from build123d import *

# Parameters (mm, degrees)
SKETCH_1_R      = 4
EXTRUDE_1_DEPTH = 13
SKETCH_2_W      = 0.5
SKETCH_2_H      = 0.5
EXTRUDE_2_DEPTH = 1
SKETCH_3_W      = 0.5
SKETCH_3_H      = 0.5
EXTRUDE_3_DEPTH = 5.5
FILLET_1_R      = 0.25
FILLET_2_R      = 0.25


with BuildPart() as part:
    # Эскиз1 → Бобышка-Вытянуть1 (new body)
    with BuildSketch(Plane.XY):
        with Locations(Location((0, 0, 0), (0, 0, 180))):
            Circle(SKETCH_1_R)
    extrude(amount=EXTRUDE_1_DEPTH)

    # Эскиз2 → Бобышка-Вытянуть2 (add)
    with BuildSketch(Plane(origin=(0, 0, 0), x_dir=(-1, 0, 0), z_dir=(0, 0, -1))):
        with Locations((2, 0)):
            Rectangle(SKETCH_2_W, SKETCH_2_H)
        with Locations((-2, 0)):
            Rectangle(SKETCH_2_W, SKETCH_2_H)
    extrude(amount=EXTRUDE_2_DEPTH)

    # Эскиз3 → Бобышка-Вытянуть3 (add)
    with BuildSketch(Plane.XZ.offset(0.25)):
        with Locations((-2, -0.75)):
            Rectangle(SKETCH_3_W, SKETCH_3_H)
        with Locations((2, -0.75)):
            Rectangle(SKETCH_3_W, SKETCH_3_H)
    extrude(amount=EXTRUDE_3_DEPTH)

    # Скругление1
    fillet_1_edges = [part.edges().sort_by_distance(p)[0] for p in [
        (-1.75, -2.75, -1),
        (-2.25, -2.75, -1),
    ]]
    fillet(fillet_1_edges, radius=FILLET_1_R - 0.0001)  # a hair under: the kernel refuses the full size

    # Скругление2
    fillet_2_edges = [part.edges().sort_by_distance(p)[0] for p in [
        (-1.75, -0.25, -0.25),
        (-2.25, -0.25, -0.25),
        (-2.25, -3, -0.5),
        (-2, -0.25, -0.5),
        (-1.75, -3, -0.5),
        (1.75, -0.25, -0.25),
        (2.25, -0.25, -0.25),
        (1.75, -3, -0.5),
        (2, -0.25, -0.5),
        (2.25, -3, -0.5),
        (-1.75, 0.25, -0.37505),
        (-2.25, 0.25, -0.37505),
        (-2.176805985, 0.25, -0.926805985),
        (-1.823194015, 0.25, -0.926805985),
        (1.75, 0.25, -0.5),
        (2.25, 0.25, -0.5),
        (1.75, -2.75, -1),
        (2, 0.25, -1),
        (2.25, -2.75, -1),
    ]]
    fillet(fillet_2_edges, radius=FILLET_2_R - 0.0001)  # a hair under: the kernel refuses the full size


solid = part.part
Could you check a few things on this model? Use its own coordinates, in mm. Coordinates: 2 decimals unless noted, no trailing zeros. Write each loop counter-clockwise with the first axis right and the second up, starting at its lowest first coordinate (ties: lowest second). Pieces come first, ordered by that corner, then holes. Notation, with made-up numbers: (-28.5, 7.25) - (16.5, 7.25) arc R18 cw to (16.5, 23.25) - close; hole circle Ø2 at (4, 56). An arc over 180 degrees is marked (long way). Put each result on its own line as item: value. Start each with the question number.
Q1. I'm going to push flat-ended pins straight in: P1, Ø2, axis at x = 0.5, y = -1.5, coming from the -Z side; P2, Ø1.5, axis at y = 1.5, z = 5.5, coming from the -X side; P3, Ø3, axis at x = -2, z = 10, coming from the +Y side. Where does each tip first touch, or does it pass through?
Q2. I want a section at B-B on z = 2. Write out the boundary of the cut face in (x, y).
Q3. I want a section at A-A on y = -2.25. Count the separate pieces of the cut face and the enclosed holes in it, plus the area to 3 significant figures.
Q4. Please list where these lines run through material, in increasing order: L1, parallel to Z at x = -2, y = 2.5; L2, parallel to Y at x = 0, z = 12.25; L3, parallel to Y at x = -2.25, z = 5.25.
Q5. I want a section at D-D on y = 1.5. Write out the boundary of the cut face in (x, z), plus the area to 3 significant figures.
Q6. I want a section at C-C on x = 0. Write out the boundary of the cut face in (y, z), plus the area to 3 significant figures.
Checks:
1. P1: z = 0
1. P2: x = -3.93
1. P3: y = 3.97
2. outline: circle Ø8 at (0, 0)
3. separate pieces: 3
3. enclosed holes: 0
3. area: 86.4 mm²
4. L1: 0 to 13
4. L2: -4 to 4
4. L3: -3.31 to 3.31
5. outline: (-3.71, 0) - (3.71, 0) - (3.71, 13) - (-3.71, 13) - close
5. area: 96.4 mm²
6. outline: (-4, 0) - (4, 0) - (4, 13) - (-4, 13) - close
6. area: 104 mm²
